Read the model definition and answer for the solid it produces. Units are mm, in the model's axes. A direction names the side the tool comes from. Round coordinates to 2 decimals unless told otherwise and drop trailing zeros. Write each loop counter-clockwise with the first axis right and the second up, starting at its lowest first coordinate (ties: lowest second). Pieces come first, ordered by that corner, then holes. Notation, with made-up numbers: (-15, 6) - (39, 6) arc R11 ccw to (39, 10) - close; hole circle Ø11 at (-3, 27). An arc over 180 degrees is marked (long way). One line per item, written item: value. Start each with the question number.
(1) Flat-ended cylindrical pins translate along their axes: pin 1 Ø4 at (y, z) = (16, -8.5) entering from +X; pin 2 Ø2 at (y, z) = (0, 0) entering from -X; pin 3 Ø1.3 at (y, z) = (0, 0) entering from +X; pin 4 Ø1 at (x, y) = (4, 50.5) entering from +Z. Find the tip coordinate at first contact, or state that the pin passes through.
(2) A cutting plane is placed at B-B, the plane y = 0. Determine the outline of the cut face in (x, z).
(3) For faces 5 (the face through (-14.3, 1, 0)), 6 (the face through (1.94, 3.56, -4.69)), 7 (the face through (13.6, 1, 0)), 8 (the face through (3.955, 63.68, 5.158)), determine the directions among +Z, -Z, +X, -X, +Y, -Y from which every point of the face is accessible in a straight line to the end or side of a thin tool.
(4) Find the intervals of material crossed by L1, parallel to X at y = 54, z = 0; L2, parallel to Y at x = -13.95, z = 0; L3, parallel to Y at x = 1.5, z = 5, in increasing order.
(5) A cutting plane is placed at D-D, the plane y = 59. Determine the outline of the cut face in (x, z).
(6) A cutting plane is placed at A-A, the plane x = 0. Determine the outline of the cut face in (y, z) (3 decimals).
(7) A cutting plane is placed at C-C, the plane y = 10. Determine the outline of the cut face in (x, z).
(8) The mould has two halves that part along X. Classify faces 1 (the face through (-0.785, 59.014, 17.833)), 2 (the face through (0, 2.6, 2)), 3 (the face through (-12.7, 52.38, -0.08)), 4 (the face through (6, 58, 17)): +X half, -X half, draft (parallel to the pull), parting line (faces both ways), or undercut.
from build123d import *

# Parameters (mm, degrees)
ENL_V_MAT_EXTRU_1_DEPTH                   = 15
TROU_TARAUD_M31_D                         = 2.5
TROU_TARAUD_M31_DEPTH                     = 8.5
TROU_TARAUD_M31_TIP                       = 0.751075774
ESQUISSE5_W                               = 0.7
ESQUISSE5_H                               = 3.8
BOSS_EXTRU_1_DEPTH                        = 6.7
CHANFREIN1_SIZE                           = 1
ESQUISSE6_R                               = 0.8
ENL_V_MAT_EXTRU_2_DEPTH                   = 6.7
R_P_TITION_CIRCULAIRE1_COUNT              = 2
CHANFREIN1_OF_R_P_TITION_CIRCULAIRE1_SIZE = 1
ESQUISSE7_R                               = 1.6
ENL_V_MAT_EXTRU_3_DEPTH                   = 90.145947749


with BuildPart() as part:
    # Esquisse1 → Révolution1 (revolve)
    with BuildSketch(Plane.XY, mode=Mode.PRIVATE) as r_volution1_sk:
        with BuildLine():
            Line((0, 0), (-1.6, 0))
            Line((-1.6, 0), (-1.6, 2.6))
            Line((-1.6, 2.6), (-5.075, 2.6))
            Line((-5.075, 2.6), (-5.075, 4.5))
            Line((-5.075, 4.5), (-19, 4.5))
            Line((-19, 4.5), (-19, 58))
            Line((-19, 58), (-17.85, 58))
            Line((-17.85, 58), (-17.85, 60))
            ThreePointArc((-17.85, 60), (-17.410660172, 61.060660172), (-16.35, 61.5))
            Line((-16.35, 61.5), (-6.5, 61.5))
            Line((-6.5, 61.5), (-6.5, 65.8))
            Line((-6.5, 65.8), (-1.6, 65.8))
            Line((-1.6, 65.8), (-1.6, 85))
            Line((-1.6, 85), (0, 85))
            Line((0, 85), (0, 0))
        make_face()
    revolve(r_volution1_sk.sketch.rotate(Axis((0, 0, 0), (0, 1, 0)), 270), axis=Axis((0, 0, 0), (0, 1, 0)))

    # Esquisse2 → Enlèv. mat.-Extru.1 (cut)
    with BuildSketch(Plane(origin=(0, 85, 0), x_dir=(1, 0, 0), z_dir=(0, 1, 0))):
        with BuildLine():
            Line((-1.161895004, -1.1), (1.161895004, -1.1))
            ThreePointArc((1.161895004, -1.1), (0, -1.6), (-1.161895004, -1.1))
        make_face()
    extrude(amount=-ENL_V_MAT_EXTRU_1_DEPTH, mode=Mode.SUBTRACT)

    # Trou taraudé M31
    with Locations(Plane(origin=(0, 61.5, 0), x_dir=(-1, 0, 0), z_dir=(0, 1, 0))):
        with Locations((12.5, 0), (-12.5, 0)):
            Hole(TROU_TARAUD_M31_D / 2, depth=TROU_TARAUD_M31_DEPTH)
            with Locations((0, 0, -(TROU_TARAUD_M31_DEPTH + TROU_TARAUD_M31_TIP / 2))):  # 118° drill point
                Cone(0, TROU_TARAUD_M31_D / 2, TROU_TARAUD_M31_TIP, mode=Mode.SUBTRACT)

    # Esquisse5 → Boss.-Extru.1 (add)
    with BuildSketch(Plane.XZ.offset(-4.5)):
        with Locations((-13.95, 0)):
            Rectangle(ESQUISSE5_W, ESQUISSE5_H)
    boss_extru_1 = extrude(amount=BOSS_EXTRU_1_DEPTH)

    # Chanfrein1
    chanfrein1_edges = [part.edges().sort_by_distance(p)[0] for p in [
        (-13.95, -2.2, -1.9),
        (-13.95, -2.2, 1.9),
    ]]
    chamfer(chanfrein1_edges, length=CHANFREIN1_SIZE)

    # Esquisse6 → Enlèv. mat.-Extru.2 (cut)
    with BuildSketch(Plane.ZY.offset(14.3)):
        Circle(ESQUISSE6_R)
    enl_v_mat_extru_2 = extrude(amount=-ENL_V_MAT_EXTRU_2_DEPTH, mode=Mode.SUBTRACT)

    # Répétition circulaire1: Boss.-Extru.1, Enlèv. mat.-Extru.2 ×2 about axis
    r_p_tition_circulaire1_axis = Axis((0, 0, 0), (0, 1, 0))
    add([boss_extru_1.rotate(r_p_tition_circulaire1_axis, i * 360 / R_P_TITION_CIRCULAIRE1_COUNT) for i in range(1, R_P_TITION_CIRCULAIRE1_COUNT)])
    add([enl_v_mat_extru_2.rotate(r_p_tition_circulaire1_axis, i * 360 / R_P_TITION_CIRCULAIRE1_COUNT) for i in range(1, R_P_TITION_CIRCULAIRE1_COUNT)], mode=Mode.SUBTRACT)

    # Chanfrein1 of Répétition circulaire1
    chanfrein1_of_r_p_tition_circulaire1_edges = [part.edges().sort_by_distance(p)[0] for p in [
        (13.95, -2.2, 1.9),
        (13.95, -2.2, -1.9),
    ]]
    chamfer(chanfrein1_of_r_p_tition_circulaire1_edges, length=CHANFREIN1_OF_R_P_TITION_CIRCULAIRE1_SIZE)

    # Esquisse7 → Enlèv. mat.-Extru.3 (cut, through all)
    with BuildSketch(Plane.XZ):
        with Locations(Location((0, 0, 0), (0, 0, 270))):
            Circle(ESQUISSE7_R)
    extrude(amount=-ENL_V_MAT_EXTRU_3_DEPTH, mode=Mode.SUBTRACT)


solid = part.part
Here are the results:
1. pin 1: x = 17.85
1. pin 2: x = -14.3
1. pin 3: through
1. pin 4: z = 18.67
2. outline: (-14.3, -1.9) - (-13.6, -1.9) - (-13.6, -0.8) - (-14.3, -0.8) - close; (-14.3, 0.8) - (-13.6, 0.8) - (-13.6, 1.9) - (-14.3, 1.9) - close; (13.6, -1.9) - (14.3, -1.9) - (14.3, -0.8) - (13.6, -0.8) - close; (13.6, 0.8) - (14.3, 0.8) - (14.3, 1.9) - (13.6, 1.9) - close
3. face 5: +Z, -Z, -X, -Y
3. face 6: -Y
3. face 7: +Z, -Z, -Y
3. face 8: +Y
4. L1: -19 to -13.75, -11.25 to -1.6, 1.6 to 11.25, 13.75 to 19
4. L2: -2.2 to -0.8, 0.8 to 61.5
4. L3: 4.5 to 65.8
5. outline: circle Ø35.7 at (0, 0); hole circle Ø2.5 at (-12.5, 0); hole circle Ø3.2 at (0, 0); hole circle Ø2.5 at (12.5, 0)
6. outline: (2.6, -5.075) - (4.5, -5.075) - (4.5, -19) - (58, -19) - (58, -17.85) - (60, -17.85) arc R1.5 ccw to (61.5, -16.35) - (61.5, -6.5) - (65.8, -6.5) - (65.8, -1.6) - (2.6, -1.6) - close; (2.6, 1.6) - (65.8, 1.6) - (65.8, 6.5) - (61.5, 6.5) - (61.5, 16.35) arc R1.5 ccw to (60, 17.85) - (58, 17.85) - (58, 19) - (4.5, 19) - (4.5, 5.075) - (2.6, 5.075) - close
7. outline: circle Ø38 at (0, 0); hole circle Ø3.2 at (0, 0)
8. face 1: parting line
8. face 2: undercut
8. face 3: undercut
8. face 4: draft
